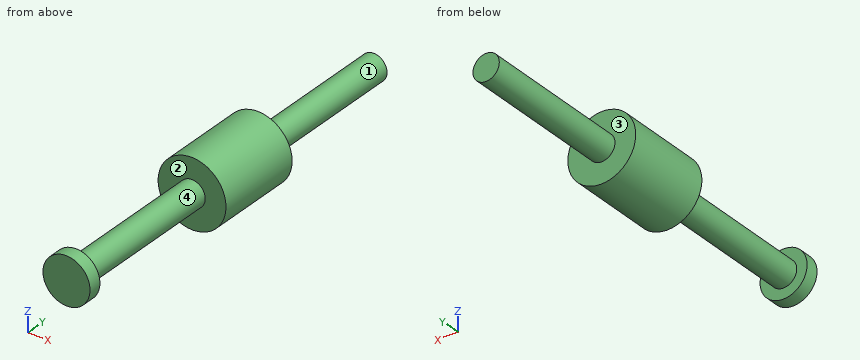
from build123d import *

# Parameters (mm, degrees)
F0_R     = 9.8054228033
F1_DEPTH = 25.4
F3_R     = 3.8049000848
F4_DEPTH = 44.45
F2_R     = 3.804929308
F5_DEPTH = 44.45
F6_R     = 6.8035972376
F7_DEPTH = 3.81


# Not quite as in the source:
# - a feature names something its author has since deleted; it is built from what else it names


with BuildPart() as f1:
    # F0 (on Front) → F1 (new body)
    with BuildSketch(Plane.XZ):
        Circle(F0_R)
    extrude(amount=F1_DEPTH)

    # F3 (on face) → F4 (join)
    with BuildSketch(Plane(origin=(0, 0, 0), x_dir=(-1, 0, 0), z_dir=(0, 1, 0))):
        Circle(F3_R)
    extrude(amount=F4_DEPTH)

    # F2 (on face) → F5 (join)
    with BuildSketch(Plane.XZ.offset(25.4)):
        Circle(F2_R)
    extrude(amount=F5_DEPTH)

    # F6 (on face) → F7 (join)
    with BuildSketch(Plane.XZ.offset(69.85)):
        Circle(F6_R)
    extrude(amount=F7_DEPTH)


solid = f1.part
The listing builds one solid part. Answer for the finished solid, in the listing's coordinates (mm). Face numbers are marked on the shaded views. Give positions to 0.01 mm unless a question says otherwise; leave off trailing zeros. Write each loop counter-clockwise with the first axis right and the second up, starting at its lowest first coordinate (ties: lowest second). Pieces come first, ordered by that corner, then holes.
1) Given P1, Ø4, axis at y = -21.5, z = -4.5, coming from the +X side; P2, Ø4, axis at x = -3, z = -2.5, coming from the +Y side; P3, Ø4, axis at x = -3, z = -6.5, coming from the +Y side; P4, Ø1.5, axis at x = 2, y = -25.5, coming from the -Z side, each flat-ended and moving along its own axis, determine where each tip first touches the part or whether it passes through.
2) Section A-A (x = 0) is taken. Write down the section's boundary in (y, z), and give its area (3 significant figures).
3) Section B-B (z = 0) is taken. Write down the section's boundary in (x, y), and give its area (3 significant figures).
4) Section D-D (y = -24) is taken. Write down the section's boundary in (x, z), and give its area (3 significant figures).
5) For a pull along Y with two mould halves and no side action, classify the marked faces 1, 2, 3 and 4 as pulls with the +Y half, pulls with the -Y half, needs draft (parallel to the pull), parting line crosses it, or undercut.
6) Find the intervals of material crossed by L1, parallel to Y at x = -5, z = 3; L2, parallel to Y at x = -5, z = 5.5; L3, parallel to Z at x = 4, y = -6, in increasing order.
7) Section C-C (y = -63) is taken. Write down the section's boundary in (x, z).
Response:
1. P1: stops at x = 9.48
1. P2: stops at y = 44.45
1. P3: stops at y = 0
1. P4: stops at z = -9.72
2. outline: (-73.66, -6.8) - (-69.85, -6.8) - (-69.85, -3.8) - (-25.4, -3.8) - (-25.4, -9.81) - (0, -9.81) - (0, -3.8) - (44.45, -3.8) - (44.45, 3.8) - (0, 3.8) - (0, 9.81) - (-25.4, 9.81) - (-25.4, 3.8) - (-69.85, 3.8) - (-69.85, 6.8) - (-73.66, 6.8) - close
2. area: 1,230 mm2
3. outline: (-9.81, -25.4) - (-3.8, -25.4) - (-3.8, -69.85) - (-6.8, -69.85) - (-6.8, -73.66) - (6.8, -73.66) - (6.8, -69.85) - (3.8, -69.85) - (3.8, -25.4) - (9.81, -25.4) - (9.81, 0) - (3.8, 0) - (3.8, 44.45) - (-3.8, 44.45) - (-3.8, 0) - (-9.81, 0) - close
3. area: 1,230 mm2
4. outline: circle Ø19.61 at (0, 0)
4. area: 302 mm2
5. face 1: needs draft
5. face 2: undercut
5. face 3: pulls with the +Y half
5. face 4: undercut
6. L1: y = -73.66 to -69.85, -25.4 to 0
6. L2: y = -25.4 to 0
6. L3: z = -8.95 to 8.95
7. outline: circle Ø7.61 at (0, 0)
